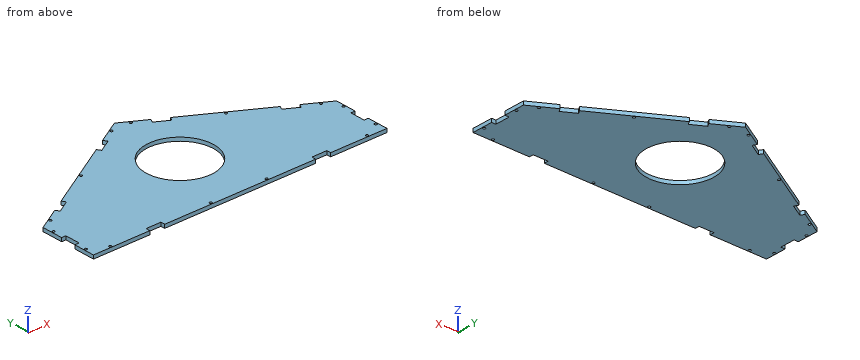
Autodesk Inventor part; units mm, degrees
ref_plane "Work Plane1" through (262.89, 0, 0) normal (-1, 0, 0) x (0, 0, 1)
ref_plane "YZ Plane" through (0, 0, 0) normal (1, 0, 0) x (0, 1, 0)
ref_plane "XZ Plane" through (0, 0, 0) normal (0, 1, 0) x (-1, 0, 0)
sketch "Sketch1" plane through (0, 0, 0) normal (0, 0, 1) x (1, 0, 0)
  line L0 (0, 0) -> (0, 101.6)
  line L1 (0, 0) -> (525.78, 0)
  line L2 (525.78, 0) -> (525.78, 101.6)
  line L3 (525.78, 101.6) -> (262.89, 253.3796)
  line L4 (262.89, 253.3796) -> (0, 101.6)
  circle A0 centre (262.89, 121.3796) radius 60
  line L5 (3.175, 99.7669) -> (3.175, 3.175) construction
  line L6 (3.175, 3.175) -> (522.605, 3.175) construction
  line L7 (522.605, 3.175) -> (522.605, 99.7669) construction
  line L8 (522.605, 99.7669) -> (262.89, 249.7134) construction
  line L9 (262.89, 249.7134) -> (3.175, 99.7669) construction
  line L10 (6.35, 97.9338) -> (6.35, 6.35) construction
  line L11 (6.35, 6.35) -> (519.43, 6.35) construction
  line L12 (519.43, 6.35) -> (519.43, 97.9338) construction
  line L13 (519.43, 97.9338) -> (262.89, 246.0473) construction
  line L14 (262.89, 246.0473) -> (6.35, 97.9338) construction
  circle A1 centre (3.175, 83.971) radius 2.25
  circle A2 centre (3.175, 18.971) radius 2.25
  line L15 (3.175, 83.971) -> (3.175, 18.971) construction
  circle A3 centre (32.89, 3.175) radius 2.25
  circle A4 centre (212.89, 3.175) radius 2.25
  circle A5 centre (312.89, 3.175) radius 2.25
  circle A6 centre (492.89, 3.175) radius 2.25
  line L16 (32.89, 3.175) -> (492.89, 3.175) construction
  line L17 (212.89, 3.175) -> (312.89, 3.175) construction
  line L18 (20.4492, 109.7402) -> (245.6158, 239.7402) construction
  circle A7 centre (20.4492, 109.7402) radius 2.25
  circle A8 centre (245.6158, 239.7402) radius 2.25
  line L19 (262.89, 0) -> (262.89, 253.3796) construction
  circle A9 centre (522.605, 83.971) radius 2.25
  circle A10 centre (522.605, 18.971) radius 2.25
  circle A11 centre (505.3308, 109.7402) radius 2.25
  circle A12 centre (280.1642, 239.7402) radius 2.25
  circle A13 centre (133.0325, 174.7402) radius 2.25
  circle A14 centre (392.7475, 174.7402) radius 2.25
  point P0 (3.175, 51.471)
  point P1 (3.175, 51.471)
  point P2 (262.89, 3.175)
  point P3 (262.89, 3.175)
  point P4 (262.89, 3.175)
  dimension "d0" = 101.6
  dimension "d1" = 525.78
  dimension "d2" = 120
  dimension "d3" = 120
  dimension "d4" = 121.3796
  dimension "d5" = 3.175
  dimension "d6" = 3.175
  dimension "d7" = 4.5
  dimension "d8" = 4.5
  dimension "d9" = 65
  dimension "d10" = 4.5
  dimension "d11" = 4.5
  dimension "d12" = 4.5
  dimension "d13" = 4.5
  dimension "d14" = 460
  dimension "d15" = 100
  dimension "d16" = 4.5
  dimension "d17" = 4.5
  dimension "d18" = 260
  dimension "d33" = 4.5
  dimension "d34" = 4.5
extrude "Extrusion1" add sketch "Sketch1" along normal blind 6.35
sketch "Sketch2" plane through (0, 0, 0) normal (0, 0, -1) x (-1, 0, 0)
  line L0 (-100.965, 7.62) -> (-127.635, 7.62)
  line L1 (-127.635, 7.62) -> (-127.635, 0)
  line L2 (-127.635, 0) -> (-100.965, 0)
  line L3 (-100.965, 0) -> (-100.965, 7.62)
  line L4 (-525.78, 0) -> (0, 0)
  line L5 (0, 0) -> (0, 101.6)
  line L6 (0, 0) -> (-525.78, 0)
  line L7 (-262.89, 0) -> (-262.89, -49.0023)
  line L8 (-424.815, 7.62) -> (-398.145, 7.62)
  line L9 (-398.145, 7.62) -> (-398.145, 0)
  line L10 (-398.145, 0) -> (-424.815, 0)
  line L11 (-424.815, 0) -> (-424.815, 7.62)
  line L12 (0, 0) -> (-525.78, 0)
  line L13 (-525.78, 0) -> (0, 0)
  line L14 (0, 101.6) -> (0, 0)
  line L15 (0, 37.465) -> (-7.62, 37.465)
  line L16 (-7.62, 37.465) -> (-7.62, 64.135)
  line L17 (-7.62, 64.135) -> (0, 64.135)
  line L18 (0, 64.135) -> (0, 37.465)
  line L19 (-525.78, 0) -> (-525.78, 101.6)
  line L20 (-525.78, 101.6) -> (-525.78, 0)
  line L21 (-525.78, 37.465) -> (-518.16, 37.465)
  line L22 (-518.16, 37.465) -> (-518.16, 64.135)
  line L23 (-518.16, 64.135) -> (-525.78, 64.135)
  line L24 (-525.78, 64.135) -> (-525.78, 37.465)
  point P0 (0, 50.8)
  point P1 (-525.78, 50.8)
  dimension "d21" = 26.67
  dimension "d22" = 7.62
  dimension "d23" = 100.965
  dimension "d26" = 7.62
  dimension "d27" = 26.67
extrude "Extrusion2" cut sketch "Sketch2" against normal through all
sketch "Sketch3" plane through (0, 0, 0) normal (0, 0, -1) x (-1, 0, 0)
  line L0 (0, 101.6) -> (-262.89, 253.3796)
  line L1 (-43.4442, 126.6825) -> (-47.2542, 120.0834)
  line L2 (-47.2542, 120.0834) -> (-70.3511, 133.4184)
  line L3 (-70.3511, 133.4184) -> (-66.5411, 140.0175)
  line L4 (-66.5411, 140.0175) -> (-43.4442, 126.6825)
  line L5 (-131.445, 177.4898) -> (-144.4004, 155.0504)
  line L6 (-262.89, 253.3796) -> (0, 101.6)
  line L7 (-219.4458, 228.2971) -> (-223.2558, 221.698)
  line L8 (-223.2558, 221.698) -> (-200.1589, 208.363)
  line L9 (-200.1589, 208.363) -> (-196.3489, 214.9621)
  line L10 (-196.3489, 214.9621) -> (-219.4458, 228.2971)
  point P0 (0, 0)
  dimension "d28" = 7.62
  dimension "d29" = 26.67
  dimension "d30" = 50.165
extrude "Extrusion3" cut sketch "Sketch3" against normal through all
ref_plane "Work Plane1" through (262.89, 0, 0) normal (-1, 0, 0) x (0, 0, 1)
mirror "Mirror1" about plane through (262.89, 0, 0) normal (-1, 0, 0) of "Extrusion3"
equation "\"d5\" = 0.5 * d19"
equation "\"d6\" = 0.5 * d19"
equation "\"d19\" = Panel_Thickness"
equation "\"d22\" = Panel_Thickness + Fit_Tolerance"
equation "\"d26\" = Panel_Thickness + Fit_Tolerance"
equation "\"d28\" = Panel_Thickness + Fit_Tolerance"
equation "\"Fit_Tolerance\" = 1.27"
equation "\"Panel_Thickness\" = 6.35"
equation "\"Tool_Dia\" = 6.35"
properties part number "BA01" material "Polyethylene, High Density"
The listing builds one solid part. Answer for the finished solid, in the listing's coordinates (mm). Coordinates: 2 decimals unless noted, no trailing zeros. Loops run counter-clockwise (first coordinate to the right, second up) from the corner with the lowest first, then second, coordinate; pieces in that order, holes last. Notation, with made-up numbers: (-4, -22.5) -> (11, -22.5) arc R26 ccw to (11, -6.5) -> close; hole circle Ø1 at (-10.75, -18). An arc over 180 degrees is marked (long way). Return JSON: item names as keys, results as strings. Group by question number.
(1) Given pin 1 Ø1.5 at (x, z) = (192, 4.5) entering from +Y; pin 2 Ø4 at (x, y) = (492.89, 3.175) entering from +Z; pin 3 Ø3 at (x, z) = (520.5, 2.5) entering from +Y; pin 4 Ø3 at (x, z) = (158, 3.5) entering from +Y, each flat-ended and moving along its own axis, determine where each tip first touches the part or whether it passes through.
(2) Find the intervals of material crossed by probe 1 along X at (y, z) = (109, 4); probe 2 along Y at (x, z) = (135, 3); probe 3 along X at (y, z) = (149, 3.5), in increasing order. Write a range as from..to.
(3) A cutting plane is placed at B-B on z = 2.75. Count the separate pieces of the cut face and the enclosed holes in it, and give its area (3 significant figures).
(4) A cutting plane is placed at A-A on y = 167. Write down the section's boundary in (x, z), and give its area (3 significant figures).
(5) A cutting plane is placed at C-C on y = 75.5. Write down the section's boundary in (x, z).
The answers:
{
 "1": {"pin 1": "stops at y = 212.88", "pin 2": "passes through", "pin 3": "stops at y = 105.51", "pin 4": "stops at y = 193.69"},
 "2": {"probe 1": "x = 12.82..18.32, 22.57..204.18, 321.6..503.21, 507.46..512.96", "probe 2": "y = 0..173.65, 175.83..179.54", "probe 3": "x = 82.1..209.63, 316.15..443.68"},
 "3": {"separate pieces": "1", "enclosed holes": "15", "area": "80,200 mm^2"},
 "4": {"outline": "(113.28, 0) -> (223.92, 0) -> (223.92, 6.35) -> (113.28, 6.35) -> close; (301.86, 0) -> (412.5, 0) -> (412.5, 6.35) -> (301.86, 6.35) -> close", "area": "1,410 mm^2"},
 "5": {"outline": "(0, 0) -> (224.22, 0) -> (224.22, 6.35) -> (0, 6.35) -> close; (301.56, 0) -> (525.78, 0) -> (525.78, 6.35) -> (301.56, 6.35) -> close"}
}
